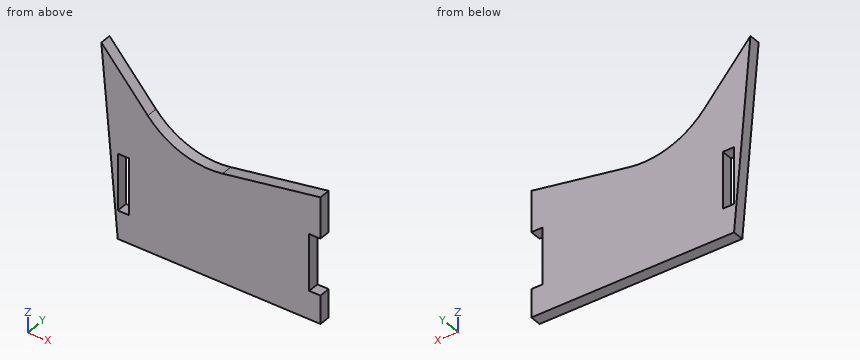
from build123d import *

# Parameters (mm, degrees)
SKETCH1_W           = 3
SKETCH1_H           = 15
BOSS_EXTRUDE1_DEPTH = 3


with BuildPart() as part:
    # Sketch1 → Boss-Extrude1 (new body)
    with BuildSketch(Plane(origin=(0, 0, 0), x_dir=(1, 0, 0), z_dir=(0, 1, 0))):
        with BuildLine():
            Line((0, 0), (-54, 0))
            Line((-54, 0), (-58.374433176, -50))
            Line((-58.374433176, -50), (-46, -35.847809072))
            ThreePointArc((-46, -35.847809072), (-36.962151982, -29.722839373), (-26.081216116, -28.82663331))
            Line((-26.081216116, -28.82663331), (0, -33.425455401))
            Line((0, -33.425455401), (0, -22.5))
            Line((0, -22.5), (-3, -22.5))
            Line((-3, -22.5), (-3, -7.5))
            Line((-3, -7.5), (0, -7.5))
            Line((0, -7.5), (0, 0))
        make_face()
        with Locations((-52.5, -15)):
            Rectangle(SKETCH1_W, SKETCH1_H, mode=Mode.SUBTRACT)
    extrude(amount=BOSS_EXTRUDE1_DEPTH)


solid = part.part
Read the model definition and answer for the solid it produces. Units are mm, in the model's axes. Coordinates: 2 decimals unless noted, no trailing zeros. Loops run counter-clockwise (first coordinate to the right, second up) from the corner with the lowest first, then second, coordinate; pieces in that order, holes last. Notation, with made-up numbers: (50.25, 13) -> (79.25, 13) arc R17 cw to (79.25, 27) -> close; hole circle Ø7 at (-34.75, 34.5). An arc over 180 degrees is marked (long way). Write item = value, one per line. Start each with the question number.
1) Given P1, Ø1.5, axis at y = 2, z = 17.5, coming from the -X side; P2, Ø0.9, axis at x = -53, y = 1, coming from the +Z side; P3, Ø5, axis at x = -46, z = 36, coming from the -Y side; P4, Ø1.5, axis at x = -1.5, y = 1.5, coming from the +Z side, each flat-ended and moving along its own axis, determine where each tip first touches the part or whether it passes through.
2) The part is cut by section D-D, the plane z = 43.5. Determine the outline of the cut face in (x, y), plus the area to 3 significant figures.
3) The part is cut by section A-A, the plane z = 12. Determine the outline of the cut face in (x, y).
4) Find the intervals of material crossed by L1, parallel to X at y = 1.05, z = 13; L2, parallel to X at y = 2.6, z = 25.5; L3, parallel to X at y = 2.65, z = 11, in increasing order. Write a range as from..to.
5) The part is cut by section B-B, the plane y = 0.75. Determine the outline of the cut face in (x, z), plus the area to 3 significant figures.
6) The part is cut by section C-C, the plane x = -53. Determine the outline of the cut face in (y, z).
Result:
q1.P1 = -55.6
q1.P2 = 44.37
q1.P3 = 0
q1.P4 = 33.29
q2.outline = (-57.81, 0) -> (-52.69, 0) -> (-52.69, 3) -> (-57.81, 3) -> close
q2.area = 15.3 mm²
q3.outline = (-55.05, 0) -> (-54, 0) -> (-54, 3) -> (-55.05, 3) -> close; (-51, 0) -> (-3, 0) -> (-3, 3) -> (-51, 3) -> close
q4.L1 = -55.14..-54, -51..-3
q4.L2 = -56.23..0
q4.L3 = -54.96..-54, -51..-3
q5.outline = (-58.37, 50) -> (-54, 0) -> (0, 0) -> (0, 7.5) -> (-3, 7.5) -> (-3, 22.5) -> (0, 22.5) -> (0, 33.43) -> (-26.08, 28.83) arc R21.5 cw to (-46, 35.85) -> close; hole (-54, 7.5) -> (-51, 7.5) -> (-51, 22.5) -> (-54, 22.5) -> close
q5.area = 1,750 mm²
q6.outline = (0, 0) -> (3, 0) -> (3, 7.5) -> (0, 7.5) -> close; (0, 22.5) -> (3, 22.5) -> (3, 43.85) -> (0, 43.85) -> close
